Read the model definition and answer for the solid it produces. Units are mm, in the model's axes. A direction names the side the tool comes from. Round coordinates to 2 decimals unless told otherwise and drop trailing zeros. Write each loop counter-clockwise with the first axis right and the second up, starting at its lowest first coordinate (ties: lowest second). Pieces come first, ordered by that corner, then holes. Notation, with made-up numbers: (38, -34) -> (92, -34) arc R16 cw to (92, -14) -> close; hole circle Ø8 at (68.25, 33). An arc over 180 degrees is marked (long way). Return JSON: item names as keys, results as strings. Group by question number.
(1) A cutting plane is placed at B-B on x = 42. Give the vertices of the cut face in (y, z), then the cut area to 3 significant figures.
(2) For faces 1 (the flat face through (-1, 16, 5.5)), 2 (the flat face through (1, -16, 5.5)), 3 (the flat face through (-1, -3, 0)), determine the directions among +Z, -Z, +X, -X, +Y, -Y from which every point of the face is accessible in a straight line to the end or side of a thin tool.
(3) Given pin 1 (4 mm diameter, centred on x = 41, z = 2.5, fed in from +Y); pin 2 (0.5 mm diameter, centred on x = -41.5, z = -0.5, fed in from +Y); pin 3 (8 mm diameter, centred on x = -65, y = 4, fed in from +Z), each flat-ended and moving along its own axis, determine where each tip first touches the part or whether it passes through.
(4) Straight lines are drawn through the part: line 1 (Y direction, x = 16, z = 5); line 2 (Z direction, x = -86.5, y = -7.5); line 3 (Z direction, x = 55, y = -16). For each, find the intervals that lie inside material, in ascending order.
(5) The mould has two halves that part along Y. Classify faces 4 (the flat face through (-100, 1.2, -0.3)), 5 (the flat face through (1, 13.5, 3)), 6 (the flat face through (1, 12.5, 3)): released by +Y, released by -Y, zero draft, split by the parting line, or undercut.
(6) A cutting plane is placed at A-A on z = 1.75. Give the vertices of the cut face in (x, y).
(7) A cutting plane is placed at C-C on y = 0. State how many separate pieces and enclosed holes the cut face has, then the cut area to 3 significant figures.
```python
from build123d import *

# Parameters (mm, degrees)
SKETCH_1_W                         = 200
SKETCH_1_H                         = 27
SM_BASE_FLANGE_1_DEPTH             = 1
SM_EDGE_FLANGE_1_STRIP_W           = 4.2
SM_EDGE_FLANGE_1_STRIP_H           = 1
SM_EDGE_FLANGE_1_STRIP_CUT_DEPTH   = 200
SM_EDGE_FLANGE_1_STRIP_2_W         = 4.2
SM_EDGE_FLANGE_1_STRIP_2_H         = 1
SM_EDGE_FLANGE_1_STRIP_CUT_2_DEPTH = 200
SM_EDGE_FLANGE_1_DEPTH             = 200
SM_EDGE_FLANGE_1_BEND_DEPTH        = 200
SM_EDGE_FLANGE_2_STRIP_W           = 4.2
SM_EDGE_FLANGE_2_STRIP_H           = 1
SM_EDGE_FLANGE_2_STRIP_CUT_DEPTH   = 200
SM_EDGE_FLANGE_2_STRIP_2_W         = 4.2
SM_EDGE_FLANGE_2_STRIP_2_H         = 1
SM_EDGE_FLANGE_2_STRIP_CUT_2_DEPTH = 200
SM_EDGE_FLANGE_2_DEPTH             = 200
SM_EDGE_FLANGE_2_BEND_DEPTH        = 200
CUT_EXTRUDE_1_DEPTH                = 10
PATTERN_LINEAR_1_COUNT             = 5
PATTERN_LINEAR_1_PITCH             = 20
PATTERN_LINEAR_1_COL_COUNT         = 5
PATTERN_LINEAR_1_COL_PITCH         = 20


# Sheet-metal steps are written as plain solids
with BuildPart() as part:
    # Sketch 1 → 基体-法兰1 (new body)
    with BuildSketch(Plane.XY):
        Rectangle(SKETCH_1_W, SKETCH_1_H)
    extrude(amount=-SM_BASE_FLANGE_1_DEPTH)

    # 边线-法兰1 strip (across the edge) → 边线-法兰1 strip cut (cut)
    with BuildSketch(Plane(origin=(100, 13.5, 0), x_dir=(0, -1, 0), z_dir=(-1, 0, 0))):
        with Locations((-1, -0.5)):
            Rectangle(SM_EDGE_FLANGE_1_STRIP_W, SM_EDGE_FLANGE_1_STRIP_H)
    extrude(amount=SM_EDGE_FLANGE_1_STRIP_CUT_DEPTH, mode=Mode.SUBTRACT)

    # 边线-法兰1 strip 2 (across the edge) → 边线-法兰1 strip cut 2 (cut)
    with BuildSketch(Plane(origin=(-100, -13.5, 0), x_dir=(0, 1, 0), z_dir=(1, 0, 0))):
        with Locations((-1, -0.5)):
            Rectangle(SM_EDGE_FLANGE_1_STRIP_2_W, SM_EDGE_FLANGE_1_STRIP_2_H)
    extrude(amount=SM_EDGE_FLANGE_1_STRIP_CUT_2_DEPTH, mode=Mode.SUBTRACT)

    # 边线-法兰1 section (across the edge) → 边线-法兰1 (add)
    with BuildSketch(Plane(origin=(100, 13.5, 0), x_dir=(0, -1, 0), z_dir=(-1, 0, 0))):
        with BuildLine():
            Line((0, 0.1), (0, 6.5))
            Line((0, 6.5), (1, 6.5))
            Line((1, 6.5), (1, 0.1))
            ThreePointArc((1, 0.1), (1.029289322, 0.029289322), (1.1, 0))
            Line((1.1, 0), (1.1, -1))
            ThreePointArc((1.1, -1), (0.322182541, -0.677817459), (0, 0.1))
        make_face()
    extrude(amount=SM_EDGE_FLANGE_1_DEPTH)

    # 边线-法兰1 section 2 (across the edge) → 边线-法兰1 bend (add)
    with BuildSketch(Plane(origin=(-100, -13.5, 0), x_dir=(0, 1, 0), z_dir=(1, 0, 0))):
        with BuildLine():
            Line((0, 0.1), (0, 6.5))
            Line((0, 6.5), (1, 6.5))
            Line((1, 6.5), (1, 0.1))
            ThreePointArc((1, 0.1), (1.029289322, 0.029289322), (1.1, 0))
            Line((1.1, 0), (1.1, -1))
            ThreePointArc((1.1, -1), (0.322182541, -0.677817459), (0, 0.1))
        make_face()
    extrude(amount=SM_EDGE_FLANGE_1_BEND_DEPTH)

    # 边线-法兰2 strip (across the edge) → 边线-法兰2 strip cut (cut)
    with BuildSketch(Plane(origin=(-100, 13.5, 6.5), x_dir=(0, 0, -1), z_dir=(1, 0, 0))):
        with Locations((-1, -0.5)):
            Rectangle(SM_EDGE_FLANGE_2_STRIP_W, SM_EDGE_FLANGE_2_STRIP_H)
    extrude(amount=SM_EDGE_FLANGE_2_STRIP_CUT_DEPTH, mode=Mode.SUBTRACT)

    # 边线-法兰2 strip 2 (across the edge) → 边线-法兰2 strip cut 2 (cut)
    with BuildSketch(Plane(origin=(100, -13.5, 6.5), x_dir=(0, 0, -1), z_dir=(-1, 0, 0))):
        with Locations((-1, -0.5)):
            Rectangle(SM_EDGE_FLANGE_2_STRIP_2_W, SM_EDGE_FLANGE_2_STRIP_2_H)
    extrude(amount=SM_EDGE_FLANGE_2_STRIP_CUT_2_DEPTH, mode=Mode.SUBTRACT)

    # 边线-法兰2 section (across the edge) → 边线-法兰2 (add)
    with BuildSketch(Plane(origin=(-100, 13.5, 6.5), x_dir=(0, 0, -1), z_dir=(1, 0, 0))):
        with BuildLine():
            Line((0, 0.1), (0, 4))
            Line((0, 4), (1, 4))
            Line((1, 4), (1, 0.1))
            ThreePointArc((1, 0.1), (1.029289322, 0.029289322), (1.1, 0))
            Line((1.1, 0), (1.1, -1))
            ThreePointArc((1.1, -1), (0.322182541, -0.677817459), (0, 0.1))
        make_face()
    extrude(amount=SM_EDGE_FLANGE_2_DEPTH)

    # 边线-法兰2 section 2 (across the edge) → 边线-法兰2 bend (add)
    with BuildSketch(Plane(origin=(100, -13.5, 6.5), x_dir=(0, 0, -1), z_dir=(-1, 0, 0))):
        with BuildLine():
            Line((0, 0.1), (0, 4))
            Line((0, 4), (1, 4))
            Line((1, 4), (1, 0.1))
            ThreePointArc((1, 0.1), (1.029289322, 0.029289322), (1.1, 0))
            Line((1.1, 0), (1.1, -1))
            ThreePointArc((1.1, -1), (0.322182541, -0.677817459), (0, 0.1))
        make_face()
    extrude(amount=SM_EDGE_FLANGE_2_BEND_DEPTH)

    # 草图18 → 切除-拉伸1 (cut)
    with BuildSketch(Plane(origin=(0, 0, -1), x_dir=(-1, 0, 0), z_dir=(0, 0, -1))):
        with BuildLine():
            Line((-4, 2.25), (4, 2.25))
            ThreePointArc((4, 2.25), (6.25, 0), (4, -2.25))
            Line((4, -2.25), (-4, -2.25))
            ThreePointArc((-4, -2.25), (-6.25, 0), (-4, 2.25))
        make_face()
    cut_extrude_1 = extrude(amount=-CUT_EXTRUDE_1_DEPTH, mode=Mode.SUBTRACT)

    # 阵列(线性)1: 切除-拉伸1 ×5
    with Locations(*[(i * PATTERN_LINEAR_1_PITCH, 0, 0) for i in range(1, PATTERN_LINEAR_1_COUNT)]):
        add(cut_extrude_1, mode=Mode.SUBTRACT)

    # 阵列(线性)1 col: 切除-拉伸1 ×5
    with Locations(*[(-i * PATTERN_LINEAR_1_COL_PITCH, 0, 0) for i in range(1, PATTERN_LINEAR_1_COL_COUNT)]):
        add(cut_extrude_1, mode=Mode.SUBTRACT)


solid = part.part
```
Checks:
{
 "1": {"outline": "(-17.5, 5.5) -> (-13.6, 5.5) arc R0.1 cw to (-13.5, 5.4) -> (-13.5, 0.1) arc R1.1 ccw to (-12.4, -1) -> (-2.25, -1) -> (-2.25, 0) -> (-12.4, 0) arc R0.1 cw to (-12.5, 0.1) -> (-12.5, 5.4) arc R1.1 ccw to (-13.6, 6.5) -> (-17.5, 6.5) -> close; (2.25, -1) -> (12.4, -1) arc R1.1 ccw to (13.5, 0.1) -> (13.5, 5.4) arc R0.1 cw to (13.6, 5.5) -> (17.5, 5.5) -> (17.5, 6.5) -> (13.6, 6.5) arc R1.1 ccw to (12.5, 5.4) -> (12.5, 0.1) arc R0.1 cw to (12.4, 0) -> (2.25, 0) -> close", "area": "42.5 mm^2"},
 "2": {"face 1": "-Z, +X, -X, +Y", "face 2": "-Z, +X, -X, -Y", "face 3": "+Z, +X, -X"},
 "3": {"pin 1": "stops at y = 13.5", "pin 2": "stops at y = 13.44", "pin 3": "stops at z = 0"},
 "4": {"line 1": "y = -13.5 to -12.5, 12.5 to 13.5", "line 2": "z = -1 to 0", "line 3": "z = 5.5 to 6.5"},
 "5": {"face 4": "zero draft", "face 5": "released by +Y", "face 6": "undercut"},
 "6": {"outline": "(-100, -13.5) -> (100, -13.5) -> (100, -12.5) -> (-100, -12.5) -> close; (-100, 12.5) -> (100, 12.5) -> (100, 13.5) -> (-100, 13.5) -> close"},
 "7": {"separate pieces": "10", "enclosed holes": "0", "area": "87.5 mm^2"}
}
